Here's how the part is built. I have some questions about the finished solid (model axes, mm). A direction names the side the tool comes from. Coordinates: 2 decimals unless noted, no trailing zeros. Order: outer loops, then holes, each group sorted by start corner. A loop starts at its lowest first (then second) coordinate and runs counter-clockwise, first axis right, second up. Notation, with made-up numbers: M 85.5,-39.75 L 113.5,-39.75 A25 cw 113.5,-6.75 Z; hole C -19,-14.75 d9. An arc over 180 degrees is marked long. Answer as CSV lines item,"result". Start each with the question number.
```python
from build123d import *

# Parameters (mm, degrees)
BOSS_EXTRUDE1_DEPTH              = 10
FILLET1_R                        = 1
SKETCH2_R                        = 0.75
BOSS_EXTRUDE2_DEPTH              = 10
BOSS_EXTRUDE3_DEPTH              = 1
F_0_55_0_55_DIAMETER_HOLE1_D     = 0.55
F_0_55_0_55_DIAMETER_HOLE1_DEPTH = 0.25
F_1_5_1_5_DIAMETER_HOLE1_D       = 1.5
F_2_0MM_DOWEL_HOLE1_D            = 2
F_2_0MM_DOWEL_HOLE1_DEPTH        = 4.499


with BuildPart() as part:
    # Sketch1 → Boss-Extrude1 (new body)
    with BuildSketch(Plane.XY):
        Polygon((0, 0), (0, 10), (2, 10), (2, 9), (5, 9), (5, 8.75), (2, 8.75), (2, 6.75), (5, 6.75), (5, 6.5), (2, 6.5), (2, 4.5), (5, 4.5), (5, 4.25), (2, 4.25), (2, 2.25), (5, 2.25), (5, 2), (2, 2), (2, 0), align=None)
    extrude(amount=BOSS_EXTRUDE1_DEPTH)

    # Fillet1
    fillet1_edges = [part.edges().sort_by_distance(p)[0] for p in [
        (1, 10, 0),
        (1, 0, 0),
        (1, 0, 10),
        (1, 10, 10),
    ]]
    fillet(fillet1_edges, radius=FILLET1_R)

    # Sketch2 → Boss-Extrude2 (add)
    with BuildSketch(Plane.XY.offset(10)):
        with Locations(Location((1, 8.871498734, 0), (0, 0, 170.134550894))):
            Circle(SKETCH2_R)
    extrude(amount=BOSS_EXTRUDE2_DEPTH)

    # Sketch3 → Boss-Extrude3 (add)
    with BuildSketch(Plane.XY.offset(14.5)):
        with BuildLine():
            Line((1, 8.871498734), (3.474873734, 11.346372468))
            ThreePointArc((3.474873734, 11.346372468), (-2.5, 8.871498734), (3.474873734, 6.396625))
            Line((3.474873734, 6.396625), (1, 8.871498734))
        make_face()
    extrude(amount=BOSS_EXTRUDE3_DEPTH)

    # Ø0.55 (0.55) Diameter Hole1
    with Locations(Plane(origin=(3.5, 9, 2), x_dir=(0, 0, 1), z_dir=(0, 1, 0))):
        with Locations((0, 0)):
            Hole(F_0_55_0_55_DIAMETER_HOLE1_D / 2, depth=F_0_55_0_55_DIAMETER_HOLE1_DEPTH)

    # Ø1.5 (1.5) Diameter Hole1 (through all)
    with Locations(Plane(origin=(0, 9, 0), x_dir=(1, 0, 0), z_dir=(0, 1, 0))):
        with Locations((3.5, -4)):
            Hole(F_1_5_1_5_DIAMETER_HOLE1_D / 2)

    # Ø2.0mm Dowel Hole1
    with Locations(Plane(origin=(0, 9, 0), x_dir=(1, 0, 0), z_dir=(0, 1, 0))):
        with Locations((3.5, -8)):
            Hole(F_2_0MM_DOWEL_HOLE1_D / 2, depth=F_2_0MM_DOWEL_HOLE1_DEPTH)


solid = part.part
```
1) Which directions (+Z, -Z, +X, -X, +Y, -Y) give clear straight access to the entire face, cutting with the end or side of a thin tool? Please do faces 1 (the face through (3, 6.75, 5)), 2 (the face through (1, 10, 5)), 3 (the face through (2, 1, 5)), 4 (the face through (2.49, 10.36, 14.99)).
2) Suppose I cut it at A-A on z = 8. Please give me the cut outline in (x, y), plus the area to 3 significant figures.
3) Suppose I cut it at D-D on y = 7.5. Please give me the cut outline in (x, z), plus the area to 3 significant figures.
4) Suppose I cut it at B-B on z = 2. Please give me the cut outline in (x, y) (3 decimals).
5) Suppose I cut it at C-C on x = 1. Please give me the cut outline in (y, z), plus the area to 3 significant figures.
6) I need wall thicknesses on line 1 (Z direction, x = 3.5, y = 6.7); line 2 (Y direction, x = 2.75, z = 2); line 3 (X direction, y = 8.8, z = 4). Which ranges of each line are inside material? Lowest first, please. Write a range as [from, to].
7) If we mould it in two halves opening along Z, with no side actions, what happens to faces 5 (the face through (1, 5, 10)), 6 (the face through (3, 2.25, 5)), 7 (the face through (1, 5, 0))? For each: released by +Z, released by -Z, zero draft, split by the parting line, or undercut.
8) Will these pins go through, and if not, where does the flat tip stop? pin 1 Ø4 at (x, y) = (4, 7) entering from -Z; pin 2 Ø2.5 at (x, z) = (3.5, 4) entering from -Y; pin 3 Ø2.5 at (x, z) = (3.5, 4) entering from +Y; pin 4 Ø1 at (y, z) = (3, 4) entering from +X.
Output:
1,face 1,"-Z, +X"
1,face 2,"-Z, +X, -X, +Y"
1,face 3,"+Z, -Z, +X, -Y"
1,face 4,"+Z, +X"
2,outline,"M 0,0 L 2,0 L 2,2 L 5,2 L 5,2.25 L 2,2.25 L 2,4.25 L 5,4.25 L 5,4.5 L 2,4.5 L 2,6.5 L 2.5,6.5 L 2.5,6.75 L 2,6.75 L 2,8.75 L 2.5,8.75 L 2.5,9 L 2,9 L 2,10 L 0,10 Z; M 4.5,6.5 L 5,6.5 L 5,6.75 L 4.5,6.75 Z; M 4.5,8.75 L 5,8.75 L 5,9 L 4.5,9 Z"
2,area,"22.0 mm²"
3,outline,"M -2.22,14.5 L 2.37,14.5 L 2.37,15.5 L -2.22,15.5 Z; M 0,0 L 2,0 L 2,10 L 0,10 Z"
3,area,"24.6 mm²"
4,outline,"M 0,0 L 2,0 L 2,2 L 5,2 L 5,2.25 L 2,2.25 L 2,4.25 L 5,4.25 L 5,4.5 L 2,4.5 L 2,6.5 L 5,6.5 L 5,6.75 L 2,6.75 L 2,8.75 L 3.225,8.75 L 3.225,9 L 2,9 L 2,10 L 0,10 Z; M 3.775,8.75 L 5,8.75 L 5,9 L 3.775,9 Z"
5,outline,"M 0,1 A1 ccw 1,0 L 9,0 A1 ccw 10,1 L 10,9 A1 ccw 9,10 L 9.62,10 L 9.62,14.5 L 12.37,14.5 L 12.37,15.5 L 9.62,15.5 L 9.62,20 L 8.12,20 L 8.12,15.5 L 5.37,15.5 L 5.37,14.5 L 8.12,14.5 L 8.12,10 L 1,10 A1 ccw 0,9 Z"
5,area,"120 mm²"
6,line 1,"[0, 3.25], [4.75, 7], [9, 10]"
6,line 2,"[2, 2.25], [4.25, 4.5], [6.5, 6.75], [8.75, 9]"
6,line 3,"[0, 2.75], [4.25, 5]"
7,face 5,"undercut"
7,face 6,"zero draft"
7,face 7,"released by -Z"
8,pin 1,"z = 0"
8,pin 2,"y = 2"
8,pin 3,"y = 9"
8,pin 4,"x = 2"
